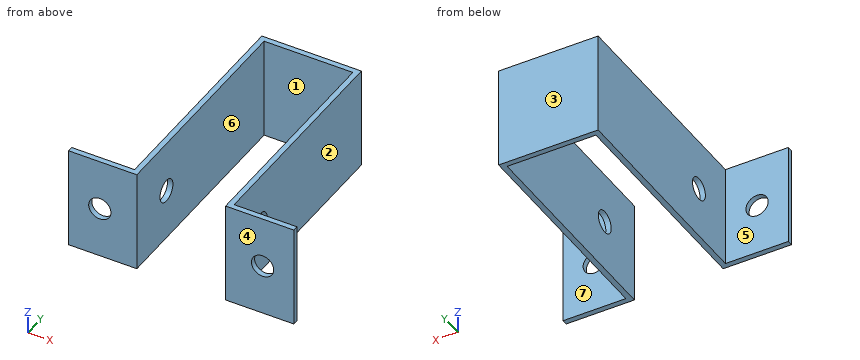
```python
from build123d import *

# Parameters (mm, degrees)
BOSS_EXTRUDE1_DEPTH   = 7.5
F_4_CLEARANCE_HOLE1_D = 3.2639
F_4_CLEARANCE_HOLE2_D = 3.2639


with BuildPart() as part:
    # Sketch1 → Boss-Extrude1 (new, symmetric)
    with BuildSketch(Plane.XY):
        Polygon((0, 32.20625), (-6.5, 32.20625), (-6.5, 0), (-16.5, 0), (-16.5, 0.79375), (-7.29375, 0.79375), (-7.29375, 33), (0, 33), align=None)
    boss_extrude1 = extrude(amount=BOSS_EXTRUDE1_DEPTH, both=True)

    # #4 Clearance Hole1 (through all)
    with Locations(Plane(origin=(-6.5, 0, 0), x_dir=(0, 0, -1), z_dir=(1, 0, 0))):
        with Locations((0, 7.5)):
            f_4_clearance_hole1 = Hole(F_4_CLEARANCE_HOLE1_D / 2)

    # Mirror1: Boss-Extrude1, #4 Clearance Hole1 across plane
    add(boss_extrude1.mirror(Plane(origin=(0, 0, 0), x_dir=(0, 0, 1), z_dir=(1, 0, 0))))
    add(f_4_clearance_hole1.mirror(Plane(origin=(0, 0, 0), x_dir=(0, 0, 1), z_dir=(1, 0, 0))), mode=Mode.SUBTRACT)

    # #4 Clearance Hole2 (through all)
    with Locations(Plane(origin=(0, 0, 0), x_dir=(-1, 0, 0), z_dir=(0, -1, 0))):
        with Locations((11.925, 0), (-11.925, 0)):
            Hole(F_4_CLEARANCE_HOLE2_D / 2)


solid = part.part
```
Check sheet for the modelled part. Datum: model origin and axes. Units: mm. Face numbers are marked on the shaded views. A direction names the side the tool comes from. Round coordinates to 2 decimals unless told otherwise and drop trailing zeros. Order: outer loops, then holes, each group sorted by start corner. A loop starts at its lowest first (then second) coordinate and runs counter-clockwise, first axis right, second up. Notation, with made-up numbers: (1, 84) -> (13, 84) arc R31 cw to (13, 123) -> close; hole circle Ø5 at (15.5, 48.25). An arc over 180 degrees is marked (long way). Use CSV: the item, a comma, the result in double quotes.
(1) Depth check by flat-ended pin: pin 1 (4 mm diameter, centred on x = 4, y = 16.5, fed in from -Z); pin 2 (4.5 mm diameter, centred on x = -11.5, z = 3, fed in from +Y); pin 3 (5 mm diameter, centred on y = 7.5, z = 0, fed in from +X); pin 4 (6.5 mm diameter, centred on x = -0.5, z = 1, fed in from -Y). Enter the tip coordinate at first touch or a pass-through.
Worked out:
pin 1,"through"
pin 2,"y = 0.79"
pin 3,"x = 7.29"
pin 4,"y = 32.21"
(2) Cross-section at A-A (y = 23). Record the boundary of the cut face in (x, z), and give its area (3 significant figures).
Worked out:
outline,"(-7.29, -7.5) -> (-6.5, -7.5) -> (-6.5, 7.5) -> (-7.29, 7.5) -> close; (6.5, -7.5) -> (7.29, -7.5) -> (7.29, 7.5) -> (6.5, 7.5) -> close"
area,"23.8 mm²"
(3) Cross-section at B-B (z = 0). Record the boundary of the cut face in (x, y).
Worked out:
outline,"(-16.5, 0) -> (-13.56, 0) -> (-13.56, 0.79) -> (-16.5, 0.79) -> close; (-10.29, 0) -> (-6.5, 0) -> (-6.5, 5.87) -> (-7.29, 5.87) -> (-7.29, 0.79) -> (-10.29, 0.79) -> close; (-7.29, 9.13) -> (-6.5, 9.13) -> (-6.5, 32.21) -> (6.5, 32.21) -> (6.5, 9.13) -> (7.29, 9.13) -> (7.29, 33) -> (-7.29, 33) -> close; (6.5, 0) -> (10.29, 0) -> (10.29, 0.79) -> (7.29, 0.79) -> (7.29, 5.87) -> (6.5, 5.87) -> close; (13.56, 0) -> (16.5, 0) -> (16.5, 0.79) -> (13.56, 0.79) -> close"
(4) Cross-section at C-C (y = 7.5). Record the boundary of the cut face in (x, z), and give its area (3 significant figures).
Worked out:
outline,"(-7.29, -7.5) -> (-6.5, -7.5) -> (-6.5, -1.63) -> (-7.29, -1.63) -> close; (-7.29, 1.63) -> (-6.5, 1.63) -> (-6.5, 7.5) -> (-7.29, 7.5) -> close; (6.5, -7.5) -> (7.29, -7.5) -> (7.29, -1.63) -> (6.5, -1.63) -> close; (6.5, 1.63) -> (7.29, 1.63) -> (7.29, 7.5) -> (6.5, 7.5) -> close"
area,"18.6 mm²"
(5) Material ranges on line 1 along X through (y, z) = (11.5, 1.5); line 2 along Y through (x, z) = (6.8, 0); line 3 along Y through (x, z) = (14, 5.5), recorded low to high. Write a range as from..to.
Worked out:
line 1,"-7.29..-6.5, 6.5..7.29"
line 2,"0..5.87, 9.13..33"
line 3,"0..0.79"
(6) Tool access check on the marked faces 4, 5, 6 and 7. Record the directions out of +Z, -Z, +X, -X, +Y, -Y that give a thin tool (end or side, any length) a straight path to the whole face; none if there is none.
Worked out:
face 4,"+Z, -Z, +X, -X, -Y"
face 5,"+Z, -Z, -X, +Y"
face 6,"+Z, -Z, -Y"
face 7,"+Z, -Z, +X, +Y"
(7) Draft check along X on the marked faces 1, 2 and 3. Enter one of: pulls with the +X half, pulls with the -X half, needs draft (parallel to the pull), parting line crosses it, or undercut.
Worked out:
face 1,"undercut"
face 2,"pulls with the +X half"
face 3,"needs draft"
(8) Cross-section at D-D (x = 11.5). Record the boundary of the cut face in (y, z).
Worked out:
outline,"(0, -7.5) -> (0.79, -7.5) -> (0.79, -1.58) -> (0, -1.58) -> close; (0, 1.58) -> (0.79, 1.58) -> (0.79, 7.5) -> (0, 7.5) -> close"
